```python
from build123d import *

# Parameters (mm, degrees)
F0_R     = 50.8
F1_DEPTH = 3.175


with BuildPart() as f1:
    # F0 (on Top) → F1 (new body)
    with BuildSketch(Plane.XY):
        Circle(F0_R)
        with BuildLine():
            Line((-21.59, -37.394977), (-6.35, -10.998523))
            ThreePointArc((-6.35, -10.998523), (-3.287002, -12.267258), (0, -12.7))
            Line((0, -12.7), (0, -43.18))
            ThreePointArc((0, -43.18), (-11.175806, -41.708677), (-21.59, -37.394977))
        make_face(mode=Mode.SUBTRACT)
        with BuildLine():
            Line((-43.18, 0), (-12.7, 0))
            ThreePointArc((-12.7, 0), (-12.267258, -3.287002), (-10.998523, -6.35))
            Line((-10.998523, -6.35), (-37.394977, -21.59))
            ThreePointArc((-37.394977, -21.59), (-41.708677, -11.175806), (-43.18, 0))
        make_face(mode=Mode.SUBTRACT)
        with BuildLine():
            ThreePointArc((-1.5875, 0), (0, 1.5875), (1.5875, 0))
            ThreePointArc((1.5875, 0), (0, -1.5875), (-1.5875, 0))
        make_face(mode=Mode.SUBTRACT)
        with BuildLine():
            Line((10.998523, -6.35), (37.394977, -21.59))
            ThreePointArc((37.394977, -21.59), (30.532871, -30.532871), (21.59, -37.394977))
            Line((21.59, -37.394977), (6.35, -10.998523))
            ThreePointArc((6.35, -10.998523), (8.980256, -8.980256), (10.998523, -6.35))
        make_face(mode=Mode.SUBTRACT)
        with BuildLine():
            ThreePointArc((-37.394977, 21.59), (-30.532871, 30.532871), (-21.59, 37.394977))
            Line((-21.59, 37.394977), (-6.35, 10.998523))
            ThreePointArc((-6.35, 10.998523), (-8.980256, 8.980256), (-10.998523, 6.35))
            Line((-10.998523, 6.35), (-37.394977, 21.59))
        make_face(mode=Mode.SUBTRACT)
        with BuildLine():
            ThreePointArc((12.7, 0), (12.267258, 3.287002), (10.998523, 6.35))
            Line((10.998523, 6.35), (37.394977, 21.59))
            ThreePointArc((37.394977, 21.59), (41.708677, 11.175806), (43.18, 0))
            Line((43.18, 0), (12.7, 0))
        make_face(mode=Mode.SUBTRACT)
        with BuildLine():
            Line((0, 12.7), (0, 43.18))
            ThreePointArc((0, 43.18), (11.175806, 41.708677), (21.59, 37.394977))
            Line((21.59, 37.394977), (6.35, 10.998523))
            ThreePointArc((6.35, 10.998523), (3.287002, 12.267258), (0, 12.7))
        make_face(mode=Mode.SUBTRACT)
    extrude(amount=F1_DEPTH)


solid = f1.part
```
Input: part model. Units: mm. Frame: model coordinates. Coordinates: 2 decimals unless noted, no trailing zeros. Loops run counter-clockwise (first coordinate to the right, second up) from the corner with the lowest first, then second, coordinate; pieces in that order, holes last. Notation, with made-up numbers: M 89.5,49 L 132.5,49 A23 ccw 132.5,76 Z; hole C 24.5,63.5 d4. An arc over 180 degrees is marked long. One line per item, written item: value.
(1) Line query: line 1 along X through (y, z) = (28, 1.6); line 2 along Y through (x, z) = (15, 0.55); line 3 along Y through (x, z) = (-34.5, 1). Output: solid intervals per line, ascending. Write a range as from..to.
Filled in:
line 1: -42.39..-32.87, -16.17..0, 16.17..42.39
line 2: -48.53..-25.98, -8.66..0, 8.66..25.98, 40.49..48.53
line 3: -37.29..-19.92, 0..19.92, 25.97..37.29
(2) Section C-C (x = -19). Output: boundary loops of the cut face in (y, z) (3 decimals), and give its area (3 significant figures).
Filled in:
outline: M -47.113,0 L -38.775,0 L -38.775,3.175 L -47.113,3.175 Z; M -32.909,0 L -10.97,0 L -10.97,3.175 L -32.909,3.175 Z; M 0,0 L 10.97,0 L 10.97,3.175 L 0,3.175 Z; M 32.909,0 L 47.113,0 L 47.113,3.175 L 32.909,3.175 Z
area: 176 mm^2
(3) Section B-B (y = -23). Output: boundary loops of the cut face in (x, z) (3 decimals).
Filled in:
outline: M -45.295,0 L -13.279,0 L -13.279,3.175 L -45.295,3.175 Z; M 0,0 L 13.279,0 L 13.279,3.175 L 0,3.175 Z; M 36.545,0 L 45.295,0 L 45.295,3.175 L 36.545,3.175 Z
(4) Pin query (flat end, axial travel): pin 1 (2.5 mm diameter, centred on x = 0, y = 0, fed in from -Z); pin 2 (1.5 mm diameter, centred on y = -32, z = 0.5, fed in from -X); pin 3 (1.6 mm diameter, centred on y = -28, z = 1, fed in from -X); pin 4 (1 mm diameter, centred on y = -31.5, z = 1, fed in from -X). Return the tip coordinate at first contact, or that it passes through.
Filled in:
pin 1: through
pin 2: x = -40.05
pin 3: x = -42.9
pin 4: x = -40.24
(5) Section A-A (z = 1.1). Give the number of separate pieces and of enclosed holes in the cut face, and give its area (3 significant figures).
Filled in:
separate pieces: 1
enclosed holes: 7
area: 5,420 mm^2
(6) Section D-D (x = 24). Output: boundary loops of the cut face in (y, z) (3 decimals).
Filled in:
outline: M -44.773,0 L -35.896,0 L -35.896,3.175 L -44.773,3.175 Z; M -13.856,0 L 0,0 L 0,3.175 L -13.856,3.175 Z; M 13.856,0 L 44.773,0 L 44.773,3.175 L 13.856,3.175 Z
(7) Pull-direction query (X, two-part tool) for faces 1 (the cylindrical face through (-11.012, -49.592, 1.565)), 2 (the flat face through (28, 0, 2)), 3 (the flat face through (-1, -11, 0)); classes: +X half, -X half, draft (parallel to the pull), parting line (faces both ways), or undercut.
Filled in:
face 1: parting line
face 2: undercut
face 3: draft
